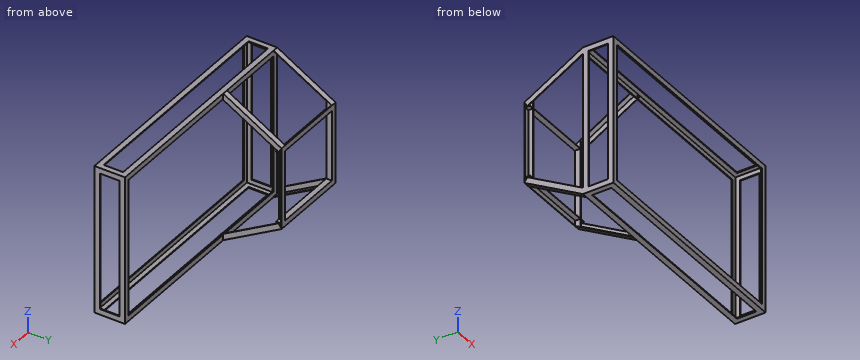
```python
from build123d import *

# Parameters (mm, degrees)
BOTTOM_HORIZONTAL_ANGLE_DEPTH   = 1574.8
BOTTOM_HORIZONTAL_ANGLE_2_DEPTH = 1574.8
BOTTOM_HORIZONTAL_ANGLE_3_DEPTH = 1574.8
BOTTOM_HORIZONTAL_ANGLE_4_DEPTH = 1574.8
FRONT_VERTIAL_ANGLE_DEPTH       = 209.55
REAR_DIAGONAL_ANGLE_DEPTH       = 460.75803
REAR_TOP_ANGLE_REACH            = 510
REAR_TOP_HORIZONTAL_ANGLE_DEPTH = 558.8
BOSS_EXTRUDE9_START             = -469.9
BOSS_EXTRUDE9_DEPTH             = 939.8


with BuildPart() as part:
    # Sketch5 → Bottom Horizontal Angle (new body)
    with BuildSketch(Plane(origin=(0, 0, 0), x_dir=(0, 0, -1), z_dir=(1, 0, 0))):
        Polygon((-508, -304.8), (-508, -266.7), (-501.65, -266.7), (-501.65, -298.45), (-469.9, -298.45), (-469.9, -304.8), align=None)
    extrude(amount=BOTTOM_HORIZONTAL_ANGLE_DEPTH)



with BuildPart() as body_2:
    # Sketch5 → Bottom Horizontal Angle 2 (new body)
    with BuildSketch(Plane(origin=(0, 0, 0), x_dir=(0, 0, -1), z_dir=(1, 0, 0))):
        Polygon((501.65, -266.7), (508, -266.7), (508, -304.8), (469.9, -304.8), (469.9, -298.45), (501.65, -298.45), align=None)
    extrude(amount=BOTTOM_HORIZONTAL_ANGLE_2_DEPTH)


with BuildPart() as body_3:
    # Sketch5 → Bottom Horizontal Angle 3 (new body)
    with BuildSketch(Plane(origin=(0, 0, 0), x_dir=(0, 0, -1), z_dir=(1, 0, 0))):
        Polygon((508, -95.25), (508, -133.35), (501.65, -133.35), (501.65, -101.6), (469.9, -101.6), (469.9, -95.25), align=None)
    extrude(amount=BOTTOM_HORIZONTAL_ANGLE_3_DEPTH)


with BuildPart() as body_4:
    # Sketch5 → Bottom Horizontal Angle 4 (new body)
    with BuildSketch(Plane(origin=(0, 0, 0), x_dir=(0, 0, -1), z_dir=(1, 0, 0))):
        Polygon((-501.65, -133.35), (-508, -133.35), (-508, -95.25), (-469.9, -95.25), (-469.9, -101.6), (-501.65, -101.6), align=None)
    extrude(amount=BOTTOM_HORIZONTAL_ANGLE_4_DEPTH)


with BuildPart() as part_1:
    add(part.part)

    add(body_2.part)  # Front Vertial Angle merges body 2

    add(body_3.part)  # Front Vertial Angle merges body 3

    add(body_4.part)  # Front Vertial Angle merges body 4
    # Sketch6 → Front Vertial Angle (add)
    with BuildSketch(Plane.XZ.offset(304.8)):
        Polygon((1574.8, -508), (1536.7, -508), (1536.7, -501.65), (1568.45, -501.65), (1568.45, -469.9), (1574.8, -469.9), align=None)
        Polygon((1536.7, 501.65), (1536.7, 508), (1574.8, 508), (1574.8, 469.9), (1568.45, 469.9), (1568.45, 501.65), align=None)
        Polygon((0, 508), (38.1, 508), (38.1, 501.65), (6.35, 501.65), (6.35, 469.9), (0, 469.9), align=None)
        Polygon((38.1, -501.65), (38.1, -508), (0, -508), (0, -469.9), (6.35, -469.9), (6.35, -501.65), align=None)
    extrude(amount=-FRONT_VERTIAL_ANGLE_DEPTH)

    # Sketch13 → Rear Diagonal Angle (add)
    with BuildSketch(Plane(origin=(0, -95.25, 508), x_dir=(-1, 0, 0), z_dir=(0, -0.868243142, 0.496138938))):
        Polygon((0, 0), (0, 38.1), (-3.175, 38.1), (-3.175, 3.175), (-38.1, 3.175), (-38.1, 0), align=None)
        Polygon((-520.7, 0), (-558.8, 0), (-558.8, 38.1), (-555.625, 38.1), (-555.625, 3.175), (-520.7, 3.175), align=None)
    extrude(amount=-REAR_DIAGONAL_ANGLE_DEPTH)

    # Sketch14 → Rear Top Angle (add, up to next)
    with BuildSketch(Plane.XY, mode=Mode.PRIVATE) as rear_top_angle_sk1:
        Polygon((33.02, 266.7), (38.1, 266.7), (38.1, 304.8), (0, 304.8), (0, 299.72), (33.02, 299.72), align=None)
    rear_top_angle_tool1 = extrude(rear_top_angle_sk1.sketch, amount=REAR_TOP_ANGLE_REACH, mode=Mode.PRIVATE) - part_1.part
    add(rear_top_angle_tool1.solids().sort_by_distance((35.56, 267.238815, 0))[0])
    # Sketch14 → Rear Top Angle (add, up to next)
    with BuildSketch(Plane.XY, mode=Mode.PRIVATE) as rear_top_angle_sk2:
        Polygon((525.78, 299.72), (525.78, 266.7), (520.7, 266.7), (520.7, 304.8), (558.8, 304.8), (558.8, 299.72), align=None)
    rear_top_angle_tool2 = extrude(rear_top_angle_sk2.sketch, amount=REAR_TOP_ANGLE_REACH, mode=Mode.PRIVATE) - part_1.part
    add(rear_top_angle_tool2.solids().sort_by_distance((525.241185, 283.21, 0))[0])

    # Sketch8 → Rear Top Horizontal Angle (add)
    with BuildSketch(Plane.ZY):
        Polygon((244.475, 266.7), (241.3, 266.7), (241.3, 304.8), (279.4, 304.8), (279.4, 301.625), (244.475, 301.625), align=None)
    extrude(amount=-REAR_TOP_HORIZONTAL_ANGLE_DEPTH)

    # Sketch15 → Boss-Extrude9 (add)
    with BuildSketch(Plane.XY.offset(BOSS_EXTRUDE9_START)):
        Polygon((0, -266.7), (0, -304.8), (38.1, -304.8), (38.1, -298.45), (6.35, -298.45), (6.35, -266.7), align=None)
        Polygon((1568.45, -266.7), (1574.8, -266.7), (1574.8, -304.8), (1536.7, -304.8), (1536.7, -298.45), (1568.45, -298.45), align=None)
        Polygon((1574.8, -133.35), (1574.8, -95.25), (1536.7, -95.25), (1536.7, -101.6), (1568.45, -101.6), (1568.45, -133.35), align=None)
        Polygon((6.35, -133.35), (0, -133.35), (0, -95.25), (38.1, -95.25), (38.1, -101.6), (6.35, -101.6), align=None)
    extrude(amount=BOSS_EXTRUDE9_DEPTH)

    # Mirror 2: part across plane


with BuildPart() as part_2:
    add(part_1.part)
    add(part_1.part.mirror(Plane.XY))


solid = part_2.part
```
The listing builds one solid part. Answer for the finished solid, in the listing's coordinates (mm). Coordinates: 2 decimals unless noted, no trailing zeros. Loops run counter-clockwise (first coordinate to the right, second up) from the corner with the lowest first, then second, coordinate; pieces in that order, holes last. Notation, with made-up numbers: (74, -18.75) -> (111, -18.75) arc R5 cw to (111, -14.75) -> close; hole circle Ø1 at (44, 85.5). An arc over 180 degrees is marked (long way). Use one line per item in the form item = value. Start each with the question number.
Item 1: The part is cut by section B-B on x = 739.5. Determine the outline of the cut face in (y, z).
Item 2: Flat-ended cylindrical pins translate along their axes: pin 1 Ø11.5 at (y, z) = (281, -42) entering from -X; pin 2 Ø5 at (y, z) = (-97, -17.5) entering from -X; pin 3 Ø3 at (x, z) = (1570, 219.5) entering from +Y; pin 4 Ø10 at (x, z) = (547, 60) entering from -Y. Find the tip coordinate at first contact, or state that the pin passes through.
Item 3: Consider L1, parallel to X at y = 108.5, z = 391; L2, parallel to Z at x = 741.5, y = -100.5; L3, parallel to X at y = 129, z = 346.5 (3 decimals). Determine where each line is inside the solid, lowest interval first. Write a range as [from, to].
Item 4: The part is cut by section A-A on y = -232.5. Determine the outline of the cut face in (x, z), then the cut area to 3 significant figures.
Item 5: The part is cut by section C-C on z = 213. Count the separate pieces of the cut face and the enclosed holes in it, then the cut area to 3 significant figures.
Answer key:
q1.outline = (-304.8, -508) -> (-266.7, -508) -> (-266.7, -501.65) -> (-298.45, -501.65) -> (-298.45, -469.9) -> (-304.8, -469.9) -> close; (-304.8, 469.9) -> (-298.45, 469.9) -> (-298.45, 501.65) -> (-266.7, 501.65) -> (-266.7, 508) -> (-304.8, 508) -> close; (-133.35, -508) -> (-95.25, -508) -> (-95.25, -469.9) -> (-101.6, -469.9) -> (-101.6, -501.65) -> (-133.35, -501.65) -> close; (-133.35, 501.65) -> (-101.6, 501.65) -> (-101.6, 469.9) -> (-95.25, 469.9) -> (-95.25, 508) -> (-133.35, 508) -> close
q2.pin_1 = 33.02
q2.pin_2 = 0
q2.pin_3 = -95.25
q2.pin_4 = 299.72
q3.L1 = [0, 38.1], [520.7, 558.8]
q3.L2 = [-508, -469.9], [469.9, 508]
q3.L3 = [0, 3.175], [555.625, 558.8]
q4.outline = (0, -508) -> (38.1, -508) -> (38.1, -501.65) -> (6.35, -501.65) -> (6.35, -469.9) -> (0, -469.9) -> close; (0, 469.9) -> (6.35, 469.9) -> (6.35, 501.65) -> (38.1, 501.65) -> (38.1, 508) -> (0, 508) -> close; (1536.7, -508) -> (1574.8, -508) -> (1574.8, -469.9) -> (1568.45, -469.9) -> (1568.45, -501.65) -> (1536.7, -501.65) -> close; (1536.7, 501.65) -> (1568.45, 501.65) -> (1568.45, 469.9) -> (1574.8, 469.9) -> (1574.8, 508) -> (1536.7, 508) -> close
q4.area = 1,770 mm2
q5.separate_pieces = 6
q5.enclosed_holes = 0
q5.area = 2,500 mm2
